Read the model definition and answer for the solid it produces. Units are mm, in the model's axes. Coordinates: 2 decimals unless noted, no trailing zeros. Write each loop counter-clockwise with the first axis right and the second up, starting at its lowest first coordinate (ties: lowest second). Pieces come first, ordered by that corner, then holes. Notation, with made-up numbers: (77.5, -16) -> (85.5, -16) arc R19 cw to (85.5, -7) -> close; hole circle Ø2 at (81, -16.75). An arc over 180 degrees is marked (long way). Answer as a JSON object with one key per item and string values. Group by question number.
(1) Find section D-D (x = 44). Give the vertices of the cut face in (y, z), then the cut area to 3 significant figures.
(2) Find section B-B (z = 2.9). Count the separate pieces of the cut face and the enclosed holes in it, then the cut area to 3 significant figures.
(3) Find section A-A (x = 26). Give the vertices of the cut face in (y, z).
(4) Flat-ended cylindrical pins translate along their axes: P1, Ø0.5, axis at x = 42.5, y = 0.5, coming from the +Z side; P2, Ø1, axis at x = 31.5, z = 3.5, coming from the +Y side; P3, Ø1.5, axis at x = 28, z = 1, coming from the +Y side. Find the tip coordinate at first contact, or state that the pin passes through.
(5) Straight lines are drawn through the part: L1, parallel to Y at x = 19.5, z = 2.2; L2, parallel to Z at x = 3, y = -1.3. For each, find the intervals that lie inside material, in ascending order.
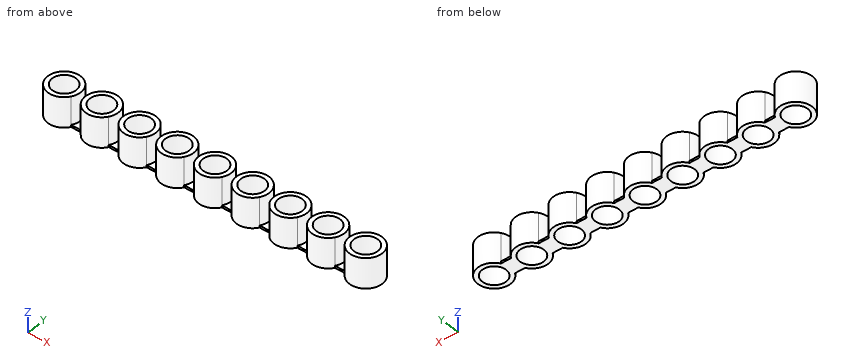
from build123d import *

# Parameters (mm, degrees)
SKETCH_R     = 2
PAD_DEPTH    = 5
POCKET_DEPTH = 4.65


with BuildPart() as part:
    # Sketch → Pad (new body)
    with BuildSketch(Plane.XY):
        with BuildLine():
            ThreePointArc((49.61843, -1.375), (54.75, 0), (49.61843, 1.375))
            Line((47.88157, 1.375), (49.61843, 1.375))
            ThreePointArc((47.88157, 1.375), (45.5, 2.75), (43.11843, 1.375))
            Line((43.11843, 1.375), (41.38157, 1.375))
            ThreePointArc((41.38157, 1.375), (39, 2.75), (36.61843, 1.375))
            Line((36.61843, 1.375), (34.88157, 1.375))
            ThreePointArc((34.88157, 1.375), (32.5, 2.75), (30.11843, 1.375))
            Line((30.11843, 1.375), (28.38157, 1.375))
            ThreePointArc((28.38157, 1.375), (26, 2.75), (23.61843, 1.375))
            Line((23.61843, 1.375), (21.88157, 1.375))
            ThreePointArc((21.88157, 1.375), (19.5, 2.75), (17.11843, 1.375))
            Line((17.11843, 1.375), (15.38157, 1.375))
            ThreePointArc((15.38157, 1.375), (13, 2.75), (10.61843, 1.375))
            Line((10.61843, 1.375), (8.88157, 1.375))
            ThreePointArc((8.88157, 1.375), (6.5, 2.75), (4.11843, 1.375))
            Line((4.11843, 1.375), (2.38157, 1.375))
            ThreePointArc((2.38157, 1.375), (-2.75, 0), (2.38157, -1.375))
            Line((2.38157, -1.375), (4.11843, -1.375))
            ThreePointArc((4.11843, -1.375), (6.5, -2.75), (8.88157, -1.375))
            Line((8.88157, -1.375), (10.61843, -1.375))
            ThreePointArc((10.61843, -1.375), (13, -2.75), (15.38157, -1.375))
            Line((15.38157, -1.375), (17.11843, -1.375))
            ThreePointArc((17.11843, -1.375), (19.5, -2.75), (21.88157, -1.375))
            Line((21.88157, -1.375), (23.61843, -1.375))
            ThreePointArc((23.61843, -1.375), (26, -2.75), (28.38157, -1.375))
            Line((28.38157, -1.375), (30.11843, -1.375))
            ThreePointArc((30.11843, -1.375), (32.5, -2.75), (34.88157, -1.375))
            Line((34.88157, -1.375), (36.61843, -1.375))
            ThreePointArc((36.61843, -1.375), (39, -2.75), (41.38157, -1.375))
            Line((41.38157, -1.375), (43.11843, -1.375))
            ThreePointArc((43.11843, -1.375), (45.5, -2.75), (47.88157, -1.375))
            Line((49.61843, -1.375), (47.88157, -1.375))
        make_face()
        Circle(SKETCH_R, mode=Mode.SUBTRACT)
        with Locations((6.5, 0)):
            Circle(SKETCH_R, mode=Mode.SUBTRACT)
        with Locations((13, 0)):
            Circle(SKETCH_R, mode=Mode.SUBTRACT)
        with Locations((19.5, 0)):
            Circle(SKETCH_R, mode=Mode.SUBTRACT)
        with Locations((26, 0)):
            Circle(SKETCH_R, mode=Mode.SUBTRACT)
        with Locations((32.5, 0)):
            Circle(SKETCH_R, mode=Mode.SUBTRACT)
        with Locations((39, 0)):
            Circle(SKETCH_R, mode=Mode.SUBTRACT)
        with Locations((45.5, 0)):
            Circle(SKETCH_R, mode=Mode.SUBTRACT)
        with Locations((52, 0)):
            Circle(SKETCH_R, mode=Mode.SUBTRACT)
    extrude(amount=PAD_DEPTH)

    # Sketch001 (on Face43 of Pad) → Pocket (cut)
    with BuildSketch(Plane.XY.offset(5)):
        with BuildLine():
            ThreePointArc((2.38157, -1.375), (2.75, 0), (2.38157, 1.375))
            Line((2.38157, 1.375), (4.11843, 1.375))
            ThreePointArc((4.11843, 1.375), (3.75, 0), (4.11843, -1.375))
            Line((4.11843, -1.375), (2.38157, -1.375))
        make_face()
        with BuildLine():
            ThreePointArc((8.88157, -1.375), (9.25, 0), (8.88157, 1.375))
            Line((8.88157, 1.375), (10.61843, 1.375))
            ThreePointArc((10.61843, 1.375), (10.25, 0), (10.61843, -1.375))
            Line((10.61843, -1.375), (8.88157, -1.375))
        make_face()
        with BuildLine():
            ThreePointArc((15.38157, -1.375), (15.75, 0), (15.38157, 1.375))
            Line((15.38157, 1.375), (17.11843, 1.375))
            ThreePointArc((17.11843, 1.375), (16.75, 0), (17.11843, -1.375))
            Line((17.11843, -1.375), (15.38157, -1.375))
        make_face()
        with BuildLine():
            ThreePointArc((23.61843, 1.375), (23.25, 0), (23.61843, -1.375))
            Line((23.61843, -1.375), (21.88157, -1.375))
            ThreePointArc((21.88157, -1.375), (22.25, 0), (21.88157, 1.375))
            Line((21.88157, 1.375), (23.61843, 1.375))
        make_face()
        with BuildLine():
            ThreePointArc((28.38157, -1.375), (28.75, 0), (28.38157, 1.375))
            Line((28.38157, 1.375), (30.11843, 1.375))
            ThreePointArc((30.11843, 1.375), (29.75, 0), (30.11843, -1.375))
            Line((30.11843, -1.375), (28.38157, -1.375))
        make_face()
        with BuildLine():
            ThreePointArc((34.88157, -1.375), (35.25, 0), (34.88157, 1.375))
            Line((34.88157, 1.375), (36.61843, 1.375))
            ThreePointArc((36.61843, 1.375), (36.25, 0), (36.61843, -1.375))
            Line((36.61843, -1.375), (34.88157, -1.375))
        make_face()
        with BuildLine():
            ThreePointArc((41.38157, -1.375), (41.75, 0), (41.38157, 1.375))
            Line((41.38157, 1.375), (43.11843, 1.375))
            ThreePointArc((43.11843, 1.375), (42.75, 0), (43.11843, -1.375))
            Line((43.11843, -1.375), (41.38157, -1.375))
        make_face()
        with BuildLine():
            ThreePointArc((47.88157, -1.375), (48.25, 0), (47.88157, 1.375))
            Line((47.88157, 1.375), (49.61843, 1.375))
            ThreePointArc((49.61843, 1.375), (49.25, 0), (49.61843, -1.375))
            Line((49.61843, -1.375), (47.88157, -1.375))
        make_face()
    extrude(amount=-POCKET_DEPTH, mode=Mode.SUBTRACT)


solid = part.part
Results below:
{
 "1": {"outline": "(-2.3, 0) -> (-1.32, 0) -> (-1.32, 5) -> (-2.3, 5) -> close; (1.32, 0) -> (2.3, 0) -> (2.3, 5) -> (1.32, 5) -> close", "area": "9.82 mm2"},
 "2": {"separate pieces": "9", "enclosed holes": "9", "area": "101 mm2"},
 "3": {"outline": "(-2.75, 0) -> (-2, 0) -> (-2, 5) -> (-2.75, 5) -> close; (2, 0) -> (2.75, 0) -> (2.75, 5) -> (2, 5) -> close"},
 "4": {"P1": "stops at z = 0.35", "P2": "stops at y = 2.7", "P3": "stops at y = 2.45"},
 "5": {"L1": "y = -2.75 to -2, 2 to 2.75", "L2": "z = 0 to 0.35"}
}
